Could you check a few things on this model? Use its own coordinates, in mm. A direction names the side the tool comes from. Give positions to 0.01 mm unless a question says otherwise; leave off trailing zeros. Loops run counter-clockwise (first coordinate to the right, second up) from the corner with the lowest first, then second, coordinate; pieces in that order, holes last.
1. Imagine slicing it at D-D (x = 12.25). List the corners of the cut face in (y, z) for me, plus the area to 3 significant figures.
2. Thinking about a two-plate mould opening in Y: for faces 4 (the cylindrical face through (8.32, 23.94, -31.41)), 5 (the flat face through (9, 15, -30)), 6 (the cylindrical face through (8.755, 15.794, -31.409)), 7 (the flat face through (-3, 0, -17)), which applies, +Y half, -Y half, draft (parallel to the pull), parting line (faces both ways), or undercut?
3. Imagine slicing it at B-B (y = 28.25). List the corners of the cut face in (x, z) for me.
4. Imagine slicing it at C-C (z = -11). List the corners of the cut face in (x, y) for me, plus the area to 3 significant figures.
5. I need wall thicknesses on line 1 along Z through (x, y) = (-8.25, 6.25); line 2 along X through (y, z) = (18.75, -15); line 3 along Z through (x, y) = (13, 12.75). Which ranges of each line are inside material? Lowest first, please.
6. For faces 1 (the flat face through (-3, 15, 0)), 2 (the flat face through (0, 16, -16)), 3 (the flat face through (3.571, 15, -15)), which set-ups out of +Z, -Z, +X, -X, +Y, -Y let a thin tool reach every point of the face, with its end or its side?
7. For P1, Ø1.7, axis at x = 8.92, y = 16.53, coming from the +Z side; P2, Ø14, axis at y = 14, z = -19, coming from the -X side; P3, Ø1.5, axis at y = 11, z = -8, coming from the +X side, each with a flat end and sliding along its axis, tell me the tip position at first contact or that it passes through.
8. Imagine slicing it at A-A (x = -4.25). List the corners of the cut face in (y, z) for me, plus the area to 3 significant figures.
```python
from build123d import *

# Parameters (mm, degrees)
BOSS_EXTRUDE1_DEPTH = 30
BOSS_EXTRUDE3_DEPTH = 10
SKETCH4_R           = 0.75
CUT_EXTRUDE1_DEPTH  = 10


with BuildPart() as part:
    # Sketch1 → Boss-Extrude1 (new body)
    with BuildSketch(Plane(origin=(0, 0, 0), x_dir=(1, 0, 0), z_dir=(0, 1, 0))):
        Polygon((0, 0), (0, 32.857142857), (14.446341209, 32.857142857), (14.446341209, 30), (3.571428571, 30), (3.571428571, 0), align=None)
    extrude(amount=BOSS_EXTRUDE1_DEPTH)

    # Sketch3 → Boss-Extrude3 (add)
    with BuildSketch(Plane.ZY):
        Polygon((-30.357142857, 0), (-32.857142857, 0), (-32.857142857, 30), (-30.357142857, 30), (-30.357142857, 27.5), (-30.357142857, 2.5), (-2.5, 2.5), (-2.5, 27.5), (-2.5, 30), (0, 30), (0, 0), (-2.5, 0), align=None)
    extrude(amount=BOSS_EXTRUDE3_DEPTH)

    # Sketch4 → Cut-Extrude1 (cut)
    with BuildSketch(Plane.XY.offset(-30)):
        with Locations((8.91712718, 24.396309317)):
            Circle(SKETCH4_R)
        with Locations((8.91712718, 16.526309317)):
            Circle(SKETCH4_R)
    extrude(amount=-CUT_EXTRUDE1_DEPTH, mode=Mode.SUBTRACT)


solid = part.part
```
Derived:
1. outline: (0, -32.86) - (30, -32.86) - (30, -30) - (0, -30) - close
1. area: 85.7 mm2
2. face 4: undercut
2. face 5: draft
2. face 6: undercut
2. face 7: -Y half
3. outline: (-10, -32.86) - (14.45, -32.86) - (14.45, -30) - (3.57, -30) - (3.57, 0) - (-10, 0) - (-10, -2.5) - (0, -2.5) - (0, -30.36) - (-10, -30.36) - close
4. outline: (-10, 0) - (3.57, 0) - (3.57, 30) - (0, 30) - (0, 2.5) - (-10, 2.5) - close
4. area: 132 mm2
5. line 1: z = -32.86 to -30.36, -2.5 to 0
5. line 2: x = 0 to 3.57
5. line 3: z = -32.86 to -30
6. face 1: +Z, +X, -X, +Y, -Y
6. face 2: -X, +Y
6. face 3: +Z, +X, +Y, -Y
7. P1: stops at z = -30
7. P2: stops at x = 0
7. P3: stops at x = 3.57
8. outline: (0, -32.86) - (30, -32.86) - (30, -30.36) - (2.5, -30.36) - (2.5, -2.5) - (30, -2.5) - (30, 0) - (0, 0) - close
8. area: 220 mm2
